For this review, take the finished solid that the model builds, in its own axes (mm). A direction names the side the tool comes from. Give positions to 0.01 mm unless a question says otherwise; leave off trailing zeros. Write each loop counter-clockwise with the first axis right and the second up, starting at its lowest first coordinate (ties: lowest second). Pieces come first, ordered by that corner, then holes.
1) Machinability: for faces 1 (the face through (0, -5, 0)), 2 (the face through (-11, 0, -27)), which of the approach directions +Z, -Z, +X, -X, +Y, -Y give a long, thin tool a straight path to every point of the face, cutting with its end or side? Answer none if there is none.
2) We need section C-C on y = 32. Give the boundary of the cut face in (x, z), and give its area (3 significant figures).
3) For P1, Ø1.5, axis at x = -15.5, z = -9, coming from the +Y side; P2, Ø1, axis at x = -8, z = -23, coming from the -Y side; P3, Ø12, axis at y = 14, z = 12, coming from the +X side; P4, Ø10, axis at y = 32, z = -18, coming from the -X side, all flat-tipped, find the tip position at first contact; note any pin that passes through.
4) Wall thickness on line 1 along Z through (x, y) = (-3.5, 22); line 2 along Z through (x, y) = (-24, 9); line 3 along X through (y, z) = (22, 9): over which ranges is each line inside the solid? List them lowest first.
5) We need section B-B on y = 3. Give the boundary of the cut face in (x, z).
from build123d import *

# Parameters (mm, degrees)
F2_R     = 28.4
F3_DEPTH = 5
F4_R     = 4.99999


# Not quite as in the source:
# - a fillet or chamfer is up to 0.001 mm smaller than in the source, because OpenCascade refuses the exact size


with BuildPart() as f1:
    # F0 (on Top) → F1 (revolve)
    with BuildSketch(Plane.XY):
        with BuildLine():
            ThreePointArc((0, 37.1231260896), (-4.3133778971, 34.6519145578), (-4.3630481141, 29.6810345364))
            ThreePointArc((-4.3630481141, 29.6810345364), (-22.7034297346, 19.6100555402), (-30, 0))
            Line((-30, 0), (0, 0))
            Line((0, 0), (0, 27.1231260896))
            Line((0, 27.1231260896), (0, 30))
            Line((0, 30), (0, 37.1231260896))
        make_face()
    revolve(axis=Axis((0, 15, 0), (0, 1, 0)))

    # F2 (on Front) → F3 (join)
    with BuildSketch(Plane.XZ):
        Circle(F2_R)
    extrude(amount=F3_DEPTH)

    # F4 (radius 5 in the source; OpenCascade refuses exactly that, so slightly less here)
    f4_edges = [f1.edges().sort_by_distance(p)[0] for p in [
        (-28.4, -5, 0),
    ]]
    fillet(f4_edges, radius=F4_R)


solid = f1.part
Results list:
1. face 1: +Z, -Z, +X, -X, -Y
1. face 2: -Y
2. outline: circle Ø10 at (0, 0)
2. area: 78.5 mm2
3. P1: stops at y = 24.6
3. P2: stops at y = -4.98
3. P3: stops at x = 27.3
3. P4: passes through
4. line 1: z = -20.09 to 20.09
4. line 2: z = -15.59 to 15.59
4. line 3: x = -18.3 to 18.3
5. outline: circle Ø59.7 at (0, 0)
